```python
from build123d import *

# Parameters (mm, degrees)
SKETCH1_W             = 30
SKETCH1_H             = 2.5
CHAMFER1_SIZE         = 0.2
CHAMFER1_SIZE2        = 0.346410162
CHAMFER1_PART_2_SIZE  = 0.2
CHAMFER1_PART_2_SIZE2 = 0.346410162


with BuildPart() as part:
    # Sketch1 → Revolve1 (revolve)
    with BuildSketch(Plane.XY):
        with Locations((-15, 1.25)):
            Rectangle(SKETCH1_W, SKETCH1_H)
    revolve(axis=Axis((0, 0, 0), (-1, 0, 0)))

    # Chamfer1
    chamfer1_edges = [part.edges().sort_by_distance(p)[0] for p in [
        (-30, -2.5, 0),
    ]]
    chamfer1_side = [part.faces().sort_by_distance(p)[0] for p in [
        (-30, 0, 0),
    ]]
    chamfer(chamfer1_edges, length=CHAMFER1_SIZE, length2=CHAMFER1_SIZE2, reference=chamfer1_side[0])

    # Chamfer1 part 2
    chamfer1_part_2_edges = [part.edges().sort_by_distance(p)[0] for p in [
        (0, -2.5, 0),
    ]]
    chamfer1_part_2_side = [part.faces().sort_by_distance(p)[0] for p in [
        (-15, -2.5, 0),
    ]]
    chamfer(chamfer1_part_2_edges, length=CHAMFER1_PART_2_SIZE, length2=CHAMFER1_PART_2_SIZE2, reference=chamfer1_part_2_side[0])


solid = part.part
```
Design review of the part built by this model. Coordinates are the model's own, in mm. Give positions to 0.01 mm unless a question says otherwise; leave off trailing zeros. Order: outer loops, then holes, each group sorted by start corner. A loop starts at its lowest first (then second) coordinate and runs counter-clockwise, first axis right, second up. Notation, with made-up numbers: M 47,13.5 L 84,13.5 A16 cw 84,17.5 Z; hole C 73.25,41 d2. An arc over 180 degrees is marked long. One line per question, with ' | ' between items. Start each with the question number.
Q1. We need section A-A (x = -12). Write out the cut boundary in (y, z).
Q2. For L1, parallel to Y at x = -8.5, z = 0.1; L2, parallel to Z at x = -7, y = -2.2; L3, parallel to Y at x = -5.25, z = -1.75, list the stretches that pass through material, from the lowest coordinate up. Write a range as [from, to].
Q3. For pin 1 Ø1.5 at (x, y) = (-7, -1) entering from -Z, flat-tipped, find the tip position at first contact; note if it passes through.
Returned:
1) outline: C 0,0 d5
2) L1: [-2.5, 2.5] | L2: [-1.19, 1.19] | L3: [-1.79, 1.79]
3) pin 1: z = -2.49
